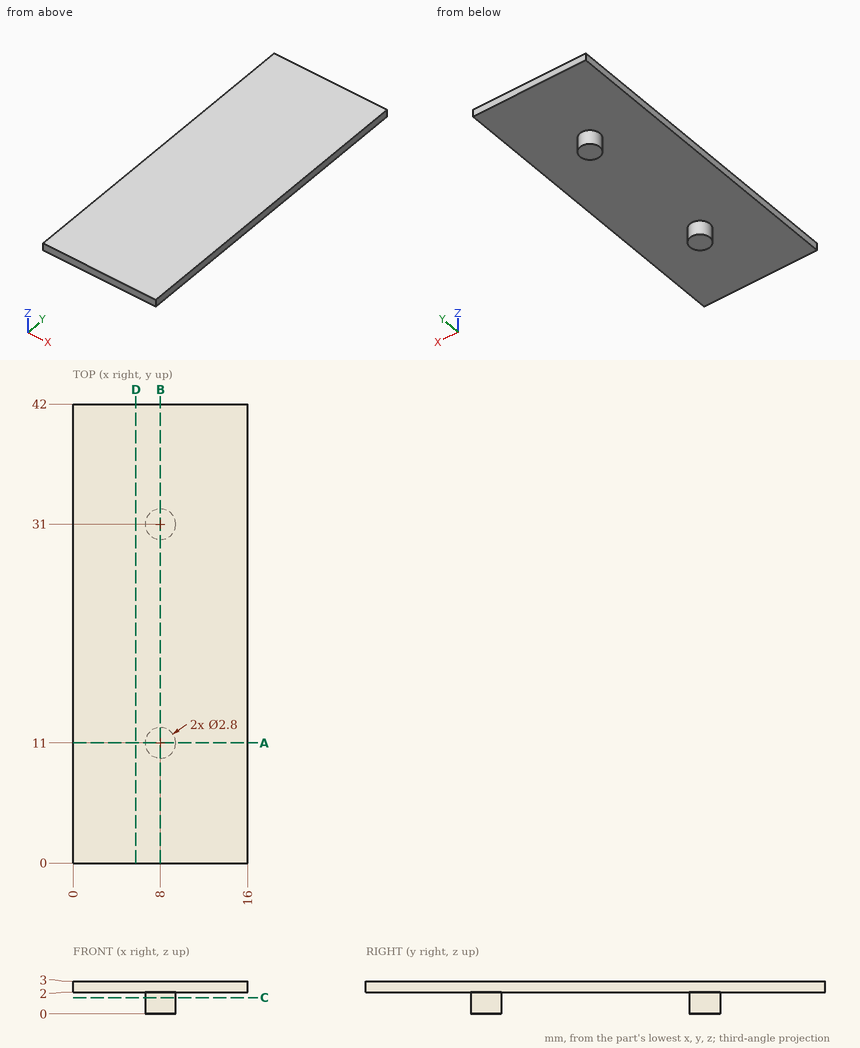
Study the drawing (mm; zero at the part's minimum x, y, z) and answer. Coordinates: 2 decimals unless noted, no trailing zeros. Write each loop counter-clockwise with the first axis right and the second up, starting at its lowest first coordinate (ties: lowest second). Pieces come first, ordered by that corner, then holes. Notation, with made-up numbers: (-34.5, -5.5) -> (-8.5, -5.5) arc R24 ccw to (-8.5, 30.5) -> close; hole circle Ø8 at (-12.5, 10.25). An arc over 180 degrees is marked (long way). Write each question's results on one line, items separated by ' | '. Start each with the question number.
1) A cutting plane is placed at D-D (x = 5.75). Determine the outline of the cut face in (y, z).
2) A flat-ended cylindrical pin translates along its axis: pin 1 Ø1.5 at (x, y) = (3.5, 20.5) entering from -Z. Find the tip coordinate at first contact, or state that the pin passes through.
3) A cutting plane is placed at A-A (y = 11). Determine the outline of the cut face in (x, z), then the cut area to 3 significant figures.
4) A cutting plane is placed at B-B (x = 8). Determine the outline of the cut face in (y, z), then the cut area to 3 significant figures.
5) A cutting plane is placed at C-C (z = 1.5). Determine the outline of the cut face in (x, y).
6) Straight lines are drawn through the part: probe 1 along Z at (x, y) = (4.25, 31); probe 2 along Y at (x, z) = (8, 1.25); probe 3 along Y at (x, z) = (9, 1.45). For each, find the intervals that lie inside material, in ascending order.
Values follow:
1) outline: (0, 2) -> (42, 2) -> (42, 3) -> (0, 3) -> close
2) pin 1: z = 2
3) outline: (0, 2) -> (6.6, 2) -> (6.6, 0) -> (9.4, 0) -> (9.4, 2) -> (16, 2) -> (16, 3) -> (0, 3) -> close | area: 21.6 mm²
4) outline: (0, 2) -> (9.6, 2) -> (9.6, 0) -> (12.4, 0) -> (12.4, 2) -> (29.6, 2) -> (29.6, 0) -> (32.4, 0) -> (32.4, 2) -> (42, 2) -> (42, 3) -> (0, 3) -> close | area: 53.2 mm²
5) outline: circle Ø2.8 at (8, 11); circle Ø2.8 at (8, 31)
6) probe 1: 2 to 3 | probe 2: 9.6 to 12.4, 29.6 to 32.4 | probe 3: 10.02 to 11.98, 30.02 to 31.98
